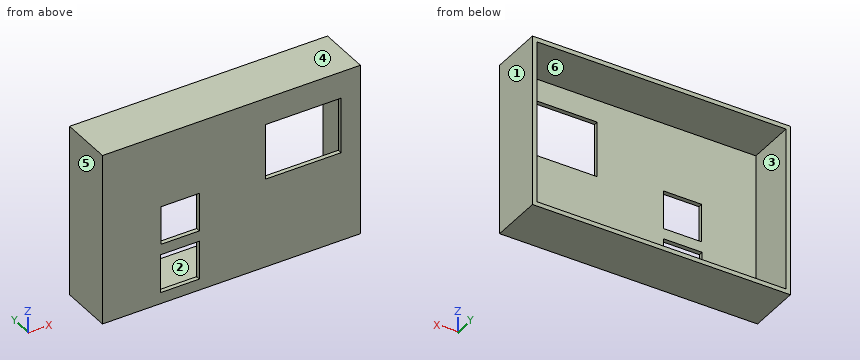
```python
from build123d import *

# Parameters (mm, degrees)
SKETCH1_W           = 150
SKETCH1_H           = 100
BOSS_EXTRUDE1_DEPTH = 30.48
SHELL1_T            = -2.54
SKETCH3_W           = 44.02563229
SKETCH3_H           = 32.399815971
CUT_EXTRUDE1_DEPTH  = 30.48
SKETCH4_W           = 22.298696875
SKETCH4_H           = 22.298696874
CUT_EXTRUDE2_DEPTH  = 30.48
SKETCH5_W           = 22.489284027
SKETCH5_H           = 22.489284027
CUT_EXTRUDE3_DEPTH  = 30.48


with BuildPart() as part:
    # Sketch1 → Boss-Extrude1 (new body)
    with BuildSketch(Plane(origin=(0, 0, 0), x_dir=(1, 0, 0), z_dir=(0, 1, 0))):
        with Locations((-34.332023576, -18.664047151)):
            Rectangle(SKETCH1_W, SKETCH1_H)
    extrude(amount=-BOSS_EXTRUDE1_DEPTH)

    # Shell1
    shell1_openings = [part.faces().sort_by_distance(p)[0] for p in [
        (-34.332023576, 0, 18.664047151),
    ]]
    offset(amount=SHELL1_T, openings=shell1_openings, kind=Kind.INTERSECTION)

    # Sketch3 → Cut-Extrude1 (cut)
    with BuildSketch(Plane.XZ.offset(30.48)):
        with Locations((7.501856458, 36.960413817)):
            Rectangle(SKETCH3_W, SKETCH3_H)
    extrude(amount=-CUT_EXTRUDE1_DEPTH, mode=Mode.SUBTRACT)

    # Sketch4 → Cut-Extrude2 (cut)
    with BuildSketch(Plane(origin=(0, -30.48, 0), x_dir=(-1, 0, 0), z_dir=(0, -1, 0))):
        with Locations((64.158912985, -14.947597672)):
            Rectangle(SKETCH4_W, SKETCH4_H)
    extrude(amount=-CUT_EXTRUDE2_DEPTH, mode=Mode.SUBTRACT)

    # Sketch5 → Cut-Extrude3 (cut)
    with BuildSketch(Plane.XZ.offset(30.48)):
        with Locations((-64.254206561, -13.545181668)):
            Rectangle(SKETCH5_W, SKETCH5_H)
    extrude(amount=-CUT_EXTRUDE3_DEPTH, mode=Mode.SUBTRACT)


solid = part.part
```
Model file for the job. Use its own axes, mm. Face numbers are marked on the shaded views. A direction names the side the tool comes from. Round coordinates to 2 decimals unless told otherwise and drop trailing zeros. Write each loop counter-clockwise with the first axis right and the second up, starting at its lowest first coordinate (ties: lowest second). Pieces come first, ordered by that corner, then holes. Notation, with made-up numbers: (-30, -13.5) -> (-2, -13.5) arc R19 cw to (-2, -9.5) -> close; hole circle Ø6 at (63.5, -34.5). An arc over 180 degrees is marked (long way). Answer as CSV lines item,"result".
1. Slice it at B-B, the plane z = 15. List the corners of the cut face in (x, y), plus the area to 3 significant figures.
Resolved:
outline,"(-109.33, -30.48) -> (-75.31, -30.48) -> (-75.31, -27.94) -> (-106.79, -27.94) -> (-106.79, 0) -> (-109.33, 0) -> close; (-53.01, -30.48) -> (40.67, -30.48) -> (40.67, 0) -> (38.13, 0) -> (38.13, -27.94) -> (-53.01, -27.94) -> close"
area,"466 mm²"
2. Slice it at C-C, the plane x = 1. List the corners of the cut face in (y, z).
Resolved:
outline,"(-30.48, -31.34) -> (0, -31.34) -> (0, -28.8) -> (-27.94, -28.8) -> (-27.94, 20.76) -> (-30.48, 20.76) -> close; (-30.48, 53.16) -> (-27.94, 53.16) -> (-27.94, 66.12) -> (0, 66.12) -> (0, 68.66) -> (-30.48, 68.66) -> close"
3. Drill centre lines: line 1 (Z direction, x = -22, y = -16); line 2 (X direction, y = -9, z = 7); line 3 (X direction, y = -29, z = 17.5). Where is each one in solid material? Low to high.
Resolved:
line 1,"-31.34 to -28.8, 66.12 to 68.66"
line 2,"-109.33 to -106.79, 38.13 to 40.67"
line 3,"-109.33 to -75.31, -53.01 to 40.67"
4. Mould opens along X. For the marked faces 3, 4, 5 and 6 say: +X half, -X half, draft (parallel to the pull), parting line (faces both ways), or undercut.
Resolved:
face 3,"undercut"
face 4,"draft"
face 5,"-X half"
face 6,"undercut"
5. Slice it at D-D, the plane x = -20. List the corners of the cut face in (y, z).
Resolved:
outline,"(-30.48, -31.34) -> (0, -31.34) -> (0, -28.8) -> (-27.94, -28.8) -> (-27.94, 66.12) -> (0, 66.12) -> (0, 68.66) -> (-30.48, 68.66) -> close"
6. Slice it at A-A, the plane y = -25.5. List the corners of the cut face in (x, z).
Resolved:
outline,"(-109.33, -31.34) -> (40.67, -31.34) -> (40.67, 68.66) -> (-109.33, 68.66) -> close; hole (-106.79, -28.8) -> (38.13, -28.8) -> (38.13, 66.12) -> (-106.79, 66.12) -> close"
7. Tool access for the marked faces 1 and 2: list every direction of +Z, -Z, +X, -X, +Y, -Y with a clear straight run to the whole face (end or side of a thin tool).
Resolved:
face 1,"+Z, -Z, +X, +Y, -Y"
face 2,"+Y"
